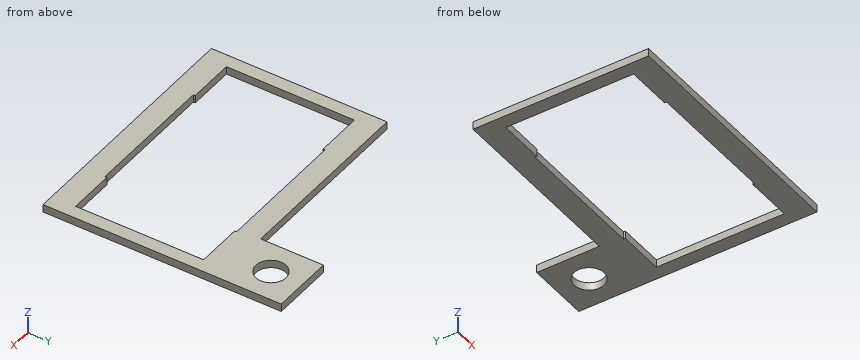
from build123d import *

# Parameters (mm, degrees)
F0_W     = 12.7
F0_H     = 12.7
F0_R     = 3.048
F1_DEPTH = 1.5875


with BuildPart() as f1:
    # F0 (on Top) → F1 (new body)
    with BuildSketch(Plane.XY):
        Polygon((-25.4, -17.78), (25.4, -17.78), (25.4, 17.78), (12.7, 17.78), (-25.4, 17.78), align=None)
        Polygon((22.733, 12.954), (22.733, -12.954), (13.335, -12.954), (13.335, -13.335), (-13.335, -13.335), (-13.335, -12.954), (-22.733, -12.954), (-22.733, 12.954), (-13.335, 12.954), (-13.335, 13.335), (13.335, 13.335), (13.335, 12.954), align=None, mode=Mode.SUBTRACT)
        with Locations((19.05, 24.13)):
            Rectangle(F0_W, F0_H)
        with Locations((19.05, 24.13)):
            Circle(F0_R, mode=Mode.SUBTRACT)
    extrude(amount=F1_DEPTH)


solid = f1.part
CAD build for the part. Positions are in the model's coordinates, mm. Round coordinates to 2 decimals unless told otherwise and drop trailing zeros. Order: outer loops, then holes, each group sorted by start corner. A loop starts at its lowest first (then second) coordinate and runs counter-clockwise, first axis right, second up. Notation, with made-up numbers: (8, -19) - (26, -19) arc R16 cw to (26, -3) - close; hole circle Ø6 at (42, -38.75). An arc over 180 degrees is marked (long way). Return JSON: item names as keys, results as strings.
(1) Cut at D-D (z = 0.8). Give the cut face in (x, y) (3 decimals).
Answer key:
{"outline": "(-25.4, -17.78) - (25.4, -17.78) - (25.4, 30.48) - (12.7, 30.48) - (12.7, 17.78) - (-25.4, 17.78) - close; hole (-22.733, -12.954) - (-13.335, -12.954) - (-13.335, -13.335) - (13.335, -13.335) - (13.335, -12.954) - (22.733, -12.954) - (22.733, 12.954) - (13.335, 12.954) - (13.335, 13.335) - (-13.335, 13.335) - (-13.335, 12.954) - (-22.733, 12.954) - close; hole circle Ø6.096 at (19.05, 24.13)"}
(2) Pin check, flat tips, straight feed: pin 1 Ø4 at (x, y) = (2, -9.5) entering from -Z; pin 2 Ø0.5 at (x, z) = (-16, 1) entering from +Y; pin 3 Ø0.8 at (y, z) = (25, 0.5) entering from -X. Stop position of each tip, or through.
Answer key:
{"pin 1": "passes through", "pin 2": "stops at y = 17.78", "pin 3": "stops at x = 12.7"}
(3) Cut at B-B (y = 24.13). Give the cut face in (x, z).
Answer key:
{"outline": "(12.7, 0) - (16, 0) - (16, 1.59) - (12.7, 1.59) - close; (22.1, 0) - (25.4, 0) - (25.4, 1.59) - (22.1, 1.59) - close"}
(4) Wall check: probe 1 along Y at (x, z) = (19.05, 0.9); probe 2 along X at (y, z) = (-8, 1.45); probe 3 along Y at (x, z) = (4, 1) (3 decimals). Give the ranges that are in metal, low to high. Write a range as from..to.
Answer key:
{"probe 1": "y = -17.78..-12.95, 12.95..21.08, 27.18..30.48", "probe 2": "x = -25.4..-22.73, 22.73..25.4", "probe 3": "y = -17.78..-13.335, 13.335..17.78"}
(5) Cut at C-C (x = 19.05). Give the cut face in (y, z).
Answer key:
{"outline": "(-17.78, 0) - (-12.95, 0) - (-12.95, 1.59) - (-17.78, 1.59) - close; (12.95, 0) - (21.08, 0) - (21.08, 1.59) - (12.95, 1.59) - close; (27.18, 0) - (30.48, 0) - (30.48, 1.59) - (27.18, 1.59) - close"}
(6) Cut at A-A (x = -1.5). Give the cut face in (y, z) (1 decimal).
Answer key:
{"outline": "(-17.8, 0) - (-13.3, 0) - (-13.3, 1.6) - (-17.8, 1.6) - close; (13.3, 0) - (17.8, 0) - (17.8, 1.6) - (13.3, 1.6) - close"}
